Can you work these out from the model? Positions are in its coordinate system, mm. A direction names the side the tool comes from. Give positions to 0.01 mm unless a question says otherwise; leave off trailing zeros. Loops run counter-clockwise (first coordinate to the right, second up) from the corner with the lowest first, then second, coordinate; pieces in that order, holes last. Notation, with made-up numbers: M 34.5,50.5 L 74.5,50.5 A18 ccw 74.5,80.5 Z; hole C 69,-3 d11. An arc over 180 degrees is marked long. Answer as a JSON object with one key per item and string values.
```python
from build123d import *

# Parameters (mm, degrees)
SKETCH_W        = 68
SKETCH_H        = 10
PAD_DEPTH       = 3
POCKET001_DEPTH = 3.001


with BuildPart() as part:
    # Sketch → Pad (new body)
    with BuildSketch(Plane.XY):
        with Locations((34, 5)):
            Rectangle(SKETCH_W, SKETCH_H)
    extrude(amount=PAD_DEPTH)

    # Sketch002 → Pocket001 (cut, through all)
    with BuildSketch(Plane.XY.offset(3)):
        with BuildLine():
            ThreePointArc((10, 7.5), (7.5, 5), (10, 2.5))
            Line((10, 2.5), (15, 2.5))
            ThreePointArc((15, 2.5), (17.5, 5), (15, 7.5))
            Line((10, 7.5), (15, 7.5))
        make_face()
        with BuildLine():
            ThreePointArc((46, 2.5), (48.5, 5), (46, 7.5))
            Line((46, 7.5), (41, 7.5))
            ThreePointArc((41, 7.5), (38.5, 5), (41, 2.5))
            Line((46, 2.5), (41, 2.5))
        make_face()
    extrude(amount=-POCKET001_DEPTH, mode=Mode.SUBTRACT)


solid = part.part
```
1) Please list where these lines run through material, in increasing order: line 1 along X through (y, z) = (5.5, 1.05); line 2 along X through (y, z) = (6, 0.95); line 3 along Y through (x, z) = (43.5, 1.9). Write a range as from..to.
Answer list:
{"line 1": "0..7.55, 17.45..38.55, 48.45..68", "line 2": "0..7.71, 17.29..38.71, 48.29..68", "line 3": "0..2.5, 7.5..10"}
2) Suppose I cut it at A-A, the plane x = 43. Write out the boundary of the cut face in (y, z).
Answer list:
{"outline": "M 0,0 L 2.5,0 L 2.5,3 L 0,3 Z; M 7.5,0 L 10,0 L 10,3 L 7.5,3 Z"}
3) For faces 4 (the cylindrical face through (7.5, 5.1, 1.5)), 5 (the flat face through (34, 5, 3)), which set-ups out of +Z, -Z, +X, -X, +Y, -Y let a thin tool reach every point of the face, with its end or its side?
Answer list:
{"face 4": "+Z, -Z", "face 5": "+Z, +X, -X, +Y, -Y"}
4) If we mould it in two halves opening along Y, with no side actions, what happens to faces 1 (the flat face through (68, 5, 1)), 2 (the flat face through (34, 10, 1)), 3 (the cylindrical face through (38.5, 5.1, 1.5))? For each: +Y half, -Y half, draft (parallel to the pull), parting line (faces both ways), or undercut.
Answer list:
{"face 1": "draft", "face 2": "+Y half", "face 3": "undercut"}
5) Suppose I cut it at B-B, the plane z = 2.2. Write out the boundary of the cut face in (x, y).
Answer list:
{"outline": "M 0,0 L 68,0 L 68,10 L 0,10 Z; hole M 10,2.5 L 15,2.5 A2.5 ccw 15,7.5 L 10,7.5 A2.5 ccw Z; hole M 41,2.5 L 46,2.5 A2.5 ccw 46,7.5 L 41,7.5 A2.5 ccw Z"}
